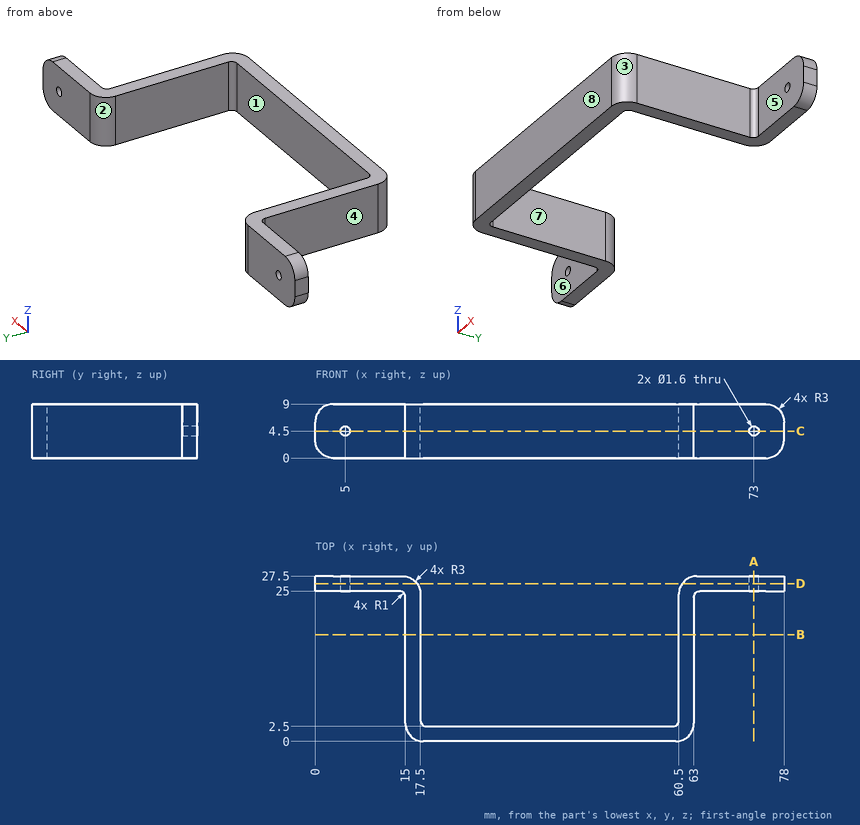
Geometry: see drawing. Coordinates: mm, zero at the bounding-box minimum. A direction names the side the tool comes from. Give positions to 0.01 mm unless a question says otherwise; leave off trailing zeros. Loops run counter-clockwise (first coordinate to the right, second up) from the corner with the lowest first, then second, coordinate; pieces in that order, holes last. Notation, with made-up numbers: (23.25, -19) -> (27.25, -19) arc R23 ccw to (27.25, 4) -> close; hole circle Ø10 at (75, 30). An arc over 180 degrees is marked (long way). Use CSV: the item, a comma, the result in double quotes.
(1) Cut plane A-A (x = 73). Output: boundary loops of the cut face in (y, z), plus the area to 3 significant figures.
From the geometry:
outline,"(25, 0) -> (27.5, 0) -> (27.5, 3.7) -> (25, 3.7) -> close; (25, 5.3) -> (27.5, 5.3) -> (27.5, 9) -> (25, 9) -> close"
area,"18.5 mm^2"
(2) Cut plane C-C (z = 4.5). Output: boundary loops of the cut face in (x, y).
From the geometry:
outline,"(0, 25) -> (4.2, 25) -> (4.2, 27.5) -> (0, 27.5) -> close; (5.8, 25) -> (14, 25) arc R1 cw to (15, 24) -> (15, 3) arc R3 ccw to (18, 0) -> (60, 0) arc R3 ccw to (63, 3) -> (63, 24) arc R1 cw to (64, 25) -> (72.2, 25) -> (72.2, 27.5) -> (63.5, 27.5) arc R3 ccw to (60.5, 24.5) -> (60.5, 3.5) arc R1 cw to (59.5, 2.5) -> (18.5, 2.5) arc R1 cw to (17.5, 3.5) -> (17.5, 24.5) arc R3 ccw to (14.5, 27.5) -> (5.8, 27.5) -> close; (73.8, 25) -> (78, 25) -> (78, 27.5) -> (73.8, 27.5) -> close"
(3) Cut plane B-B (y = 17.75). Output: boundary loops of the cut face in (x, z).
From the geometry:
outline,"(15, 0) -> (17.5, 0) -> (17.5, 9) -> (15, 9) -> close; (60.5, 0) -> (63, 0) -> (63, 9) -> (60.5, 9) -> close"
(4) Access query for the marked faces 5, 6, 7 and 8. Directions: +Z, -Z, +X, -X, +Y, -Y. A direction counts if a zero-diameter tool reaches every point of the face in a straight line with its end or side. Return the directions, or none.
From the geometry:
face 5,"+Z, -Z, +X, -Y"
face 6,"+Z, -Z, -X, -Y"
face 7,"+Z, -Z, +Y"
face 8,"+Z, -Z, +X, -X, -Y"
(5) Pull-direction query (X, two-part tool) for the marked faces 1, 2, 3 and 4; classes: released by +X, released by -X, zero draft, split by the parting line, or undercut.
From the geometry:
face 1,"undercut"
face 2,"undercut"
face 3,"released by +X"
face 4,"released by -X"
(6) First-contact query: P1, Ø4.5, axis at x = 74.5, z = 5.5, coming from the -Y side; P2, Ø2.5, axis at y = 9.5, z = 3, coming from the +X side; P3, Ø2.5, axis at x = 45.5, z = 4.5, coming from the +Y side. Flat tips, straight axial feed; report the tip coordinate or a pass-through.
From the geometry:
P1,"y = 25"
P2,"x = 63"
P3,"y = 2.5"
(7) Cut plane D-D (y = 26.25). Output: boundary loops of the cut face in (x, z).
From the geometry:
outline,"(0, 3) arc R3 ccw to (3, 0) -> (16.94, 0) -> (16.94, 9) -> (3, 9) arc R3 ccw to (0, 6) -> close; (61.06, 0) -> (75, 0) arc R3 ccw to (78, 3) -> (78, 6) arc R3 ccw to (75, 9) -> (61.06, 9) -> close; hole circle Ø1.6 at (5, 4.5); hole circle Ø1.6 at (73, 4.5)"
(8) Ray query, line 1 along X through (y, z) = (23, 0.75); line 2 along Z through (x, y) = (5, 25.7); line 3 along X through (y, z) = (26.9, 4.5). Return the intervals inside material, ascending. Write a range as [from, to].
From the geometry:
line 1,"[15, 17.5], [60.5, 63]"
line 2,"[0, 3.7], [5.3, 9]"
line 3,"[0, 4.2], [5.8, 16.3], [61.7, 72.2], [73.8, 78]"
